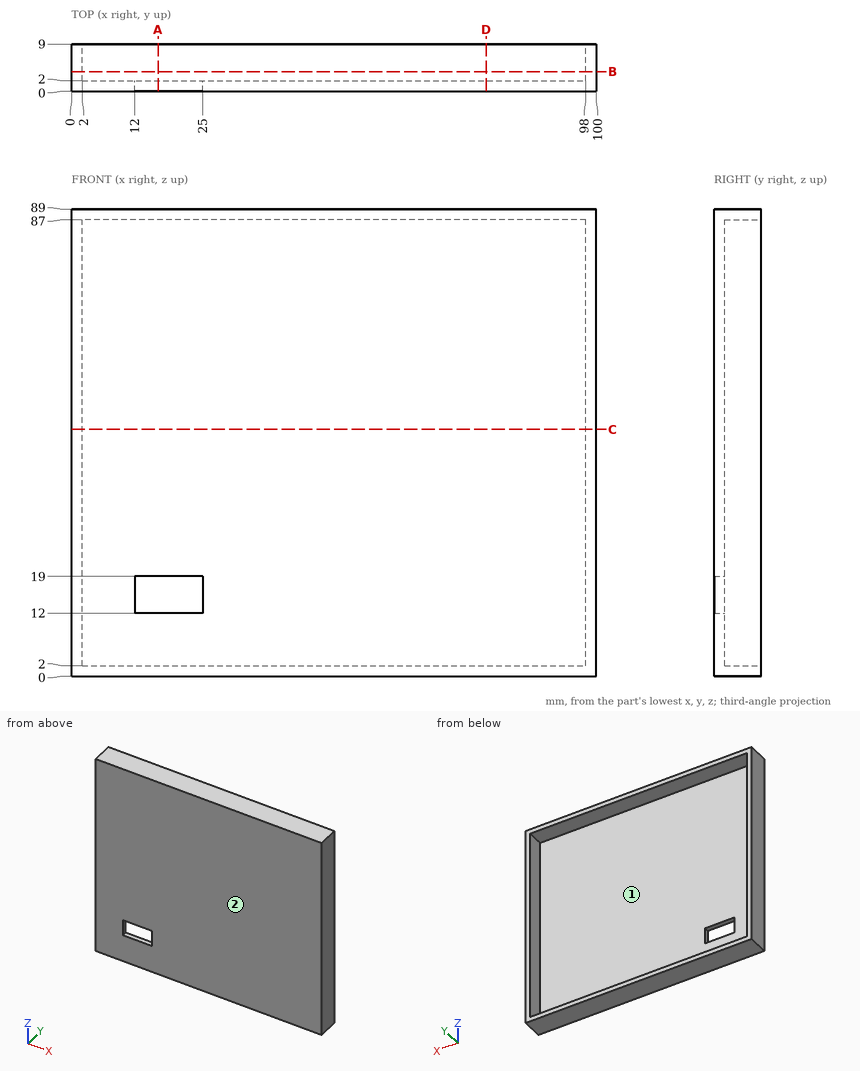
Part print with two shaded views. Sizes in mm from the minimum x, y, z corner. Round coordinates to 2 decimals unless told otherwise and drop trailing zeros. Order: outer loops, then holes, each group sorted by start corner. A loop starts at its lowest first (then second) coordinate and runs counter-clockwise, first axis right, second up. Notation, with made-up numbers: (89.25, -14.5) - (137.25, -14.5) arc R26 ccw to (137.25, 13.5) - close; hole circle Ø7 at (19, 18.5). An arc over 180 degrees is marked (long way). Return JSON: item names as keys, results as strings.
(1) Cut at C-C (z = 47). Give the cut face in (x, y), then the cut area to 3 significant figures.
Answer key:
{"outline": "(0, 0) - (100, 0) - (100, 9) - (98, 9) - (98, 2) - (2, 2) - (2, 9) - (0, 9) - close", "area": "228 mm^2"}
(2) Cut at A-A (x = 16.5). Give the cut face in (y, z), then the cut area to 3 significant figures.
Answer key:
{"outline": "(0, 0) - (9, 0) - (9, 2) - (2, 2) - (2, 12) - (0, 12) - close; (0, 19) - (2, 19) - (2, 87) - (9, 87) - (9, 89) - (0, 89) - close", "area": "192 mm^2"}
(3) Pull direction X, two halves, no side cores. Call the marked faces 1 and 2: +X half, -X half, draft (parallel to the pull), parting line (faces both ways), or undercut.
Answer key:
{"face 1": "undercut", "face 2": "draft"}
(4) Pin check, flat tips, straight feed: pin 1 Ø1 at (x, z) = (67.5, 74) entering from +Y; pin 2 Ø3.5 at (x, y) = (63.5, 5.5) entering from -Z. Stop position of each tip, or through.
Answer key:
{"pin 1": "stops at y = 2", "pin 2": "stops at z = 0"}
(5) Wall check: probe 1 along Z at (x, y) = (35, 5); probe 2 along X at (y, z) = (7.5, 11.5); probe 3 along Z at (x, y) = (13, 1.75). Give the ranges that are in metal, low to high. Write a range as from..to.
Answer key:
{"probe 1": "z = 0..2, 87..89", "probe 2": "x = 0..2, 98..100", "probe 3": "z = 0..12, 19..89"}
(6) Cut at D-D (x = 79). Give the cut face in (y, z), then the cut area to 3 significant figures.
Answer key:
{"outline": "(0, 0) - (9, 0) - (9, 2) - (2, 2) - (2, 87) - (9, 87) - (9, 89) - (0, 89) - close", "area": "206 mm^2"}
(7) Cut at B-B (y = 3.75). Give the cut face in (x, z), then the cut area to 3 significant figures.
Answer key:
{"outline": "(0, 0) - (100, 0) - (100, 89) - (0, 89) - close; hole (2, 2) - (98, 2) - (98, 87) - (2, 87) - close", "area": "740 mm^2"}
